Input: part model. Units: mm. Frame: model coordinates. A direction names the side the tool comes from. Coordinates: 2 decimals unless noted, no trailing zeros. Loops run counter-clockwise (first coordinate to the right, second up) from the corner with the lowest first, then second, coordinate; pieces in that order, holes last. Notation, with made-up numbers: (57, -3) -> (112, -3) arc R8 ccw to (112, 3) -> close; hole circle Ø6 at (77.25, 87.25). An arc over 180 degrees is marked (long way). Answer as a JSON object with one key per item and string values.
from build123d import *

# Parameters (mm, degrees)
SKETCH1_W               = 90
SKETCH1_H               = 110
BOSS_EXTRUDE2_DEPTH     = 6
SKETCH4_W               = 102
SKETCH4_H               = 122
SKETCH4_W_2             = 90
SKETCH4_H_2             = 110
BOSS_EXTRUDE3_DEPTH     = 55
SKETCH6_W               = 81.2
SKETCH6_H               = 58
SKETCH6_W_2             = 77.2
SKETCH6_H_2             = 54
BOSS_EXTRUDE4_DEPTH     = 4
CUT_EXTRUDE1_DEPTH      = 4
SKETCH12_W              = 77.2
SKETCH12_H              = 54
BOSS_EXTRUDE5_DEPTH     = 2
CUT_EXTRUDE2_REACH      = 165.966
FILLET1_R               = 2
FILLET2_R               = 2
FILLET3_R               = 2
BOSS_EXTRUDE7_DEPTH     = 4
SKETCH14_R              = 1.4
CUT_EXTRUDE3_DEPTH      = 8
MIRROR2_COPY_1_SKETCH_R = 1.4
MIRROR2_COPY_1_DEPTH    = 8


with BuildPart() as part:
    # Sketch1 → Boss-Extrude2 (new body)
    with BuildSketch(Plane(origin=(0, 0, 0), x_dir=(1, 0, 0), z_dir=(0, 1, 0))):
        with Locations((-45, 55)):
            Rectangle(SKETCH1_W, SKETCH1_H)
    extrude(amount=BOSS_EXTRUDE2_DEPTH)

    # Sketch4 → Boss-Extrude3 (add)
    with BuildSketch(Plane.XZ):
        with Locations((-45, -55)):
            Rectangle(SKETCH4_W, SKETCH4_H)
        with Locations((-45, -55)):
            Rectangle(SKETCH4_W_2, SKETCH4_H_2, mode=Mode.SUBTRACT)
    extrude(amount=-BOSS_EXTRUDE3_DEPTH)

    # Sketch6 → Boss-Extrude4 (add)
    with BuildSketch(Plane(origin=(0, 6, 0), x_dir=(1, 0, 0), z_dir=(0, 1, 0))):
        with Locations((-45, 77)):
            Rectangle(SKETCH6_W, SKETCH6_H)
        with Locations((-45, 77)):
            Rectangle(SKETCH6_W_2, SKETCH6_H_2, mode=Mode.SUBTRACT)
    extrude(amount=BOSS_EXTRUDE4_DEPTH)

    # Sketch11 → Cut-Extrude1 (cut)
    with BuildSketch(Plane(origin=(0, 10, 0), x_dir=(1, 0, 0), z_dir=(0, 1, 0))):
        Polygon((-6.4, 106), (-6.4, 104), (-6.4, 50), (-6.4, 48), (-4.4, 48), (-4.4, 106), align=None)
    extrude(amount=-CUT_EXTRUDE1_DEPTH, mode=Mode.SUBTRACT)

    # Sketch12 → Boss-Extrude5 (add)
    with BuildSketch(Plane(origin=(0, 6, 0), x_dir=(1, 0, 0), z_dir=(0, 1, 0))):
        with Locations((-45, 77)):
            Rectangle(SKETCH12_W, SKETCH12_H)
    extrude(amount=BOSS_EXTRUDE5_DEPTH)

    # Sketch10 → Cut-Extrude2 (cut, up to next)
    with BuildSketch(Plane(origin=(6, 0, 0), x_dir=(0, 0, -1), z_dir=(1, 0, 0)), mode=Mode.PRIVATE) as cut_extrude2_sk1:
        Polygon((92.5, 8), (104, 8), (104, 20.5), (92.5, 20.5), (92.5, 13.5), align=None)
    cut_extrude2_tool1 = extrude(cut_extrude2_sk1.sketch, amount=-CUT_EXTRUDE2_REACH, mode=Mode.PRIVATE) & part.part
    # Sketch10 → Cut-Extrude2 (cut, up to next)
    with BuildSketch(Plane(origin=(6, 0, 0), x_dir=(0, 0, -1), z_dir=(1, 0, 0)), mode=Mode.PRIVATE) as cut_extrude2_sk2:
        Polygon((82.5, 8), (92.5, 8), (92.5, 13.5), (82.5, 13.5), (82.5, 11.241721358), align=None)
    cut_extrude2_tool2 = extrude(cut_extrude2_sk2.sketch, amount=-CUT_EXTRUDE2_REACH, mode=Mode.PRIVATE) & part.part
    # Sketch10 → Cut-Extrude2 (cut, up to next)
    with BuildSketch(Plane(origin=(6, 0, 0), x_dir=(0, 0, -1), z_dir=(1, 0, 0)), mode=Mode.PRIVATE) as cut_extrude2_sk3:
        Polygon((65, 13.5), (65, 8), (75, 8), (75, 11.241721358), (75, 13.5), align=None)
    cut_extrude2_tool3 = extrude(cut_extrude2_sk3.sketch, amount=-CUT_EXTRUDE2_REACH, mode=Mode.PRIVATE) & part.part
    add(cut_extrude2_tool1.solids().sort_by_distance((6, 14.25, -98.25))[0], mode=Mode.SUBTRACT)
    add(cut_extrude2_tool2.solids().sort_by_distance((6, 10.75, -87.5))[0], mode=Mode.SUBTRACT)
    add(cut_extrude2_tool3.solids().sort_by_distance((6, 10.75, -70))[0], mode=Mode.SUBTRACT)

    # Fillet1
    fillet1_edges = [part.edges().sort_by_distance(p)[0] for p in [
        (6, 17, -92.5),
        (6, 13.5, -87.5),
        (6, 10.75, -82.5),
        (6, 8, -93.25),
        (6, 14.25, -104),
        (6, 20.5, -98.25),
        (6, 10.75, -65),
        (6, 8, -70),
        (6, 10.75, -75),
        (6, 13.5, -70),
    ]]
    fillet(fillet1_edges, radius=FILLET1_R)

    # Fillet2
    fillet2_edges = [part.edges().sort_by_distance(p)[0] for p in [
        (-96, 27.5, -116),
        (-96, 27.5, 6),
        (6, 27.5, 6),
        (6, 27.5, -116),
    ]]
    fillet(fillet2_edges, radius=FILLET2_R)

    # Fillet3
    fillet3_edges = [part.edges().sort_by_distance(p)[0] for p in [
        (0, 30.5, 0),
        (0, 30.5, -110),
        (-90, 30.5, -110),
        (-90, 30.5, 0),
    ]]
    fillet(fillet3_edges, radius=FILLET3_R)

    # Sketch13 → Boss-Extrude7 (add)
    with BuildSketch(Plane(origin=(0, 8, 0), x_dir=(1, 0, 0), z_dir=(0, 1, 0))):
        with BuildLine():
            ThreePointArc((-77.35, 96), (-77.862563133, 97.237436867), (-79.1, 97.75))
            Line((-79.1, 97.75), (-79.1, 96))
            Line((-79.1, 96), (-80.85, 96))
            ThreePointArc((-80.85, 96), (-79.1, 94.25), (-77.35, 96))
        make_face()
        with BuildLine():
            Line((-79.1, 96), (-79.1, 97.75))
            ThreePointArc((-79.1, 97.75), (-80.337436867, 97.237436867), (-80.85, 96))
            Line((-80.85, 96), (-79.1, 96))
        make_face()
        with BuildLine():
            ThreePointArc((-18.6, 52.25), (-17.362563133, 52.762563133), (-16.85, 54))
            Line((-16.85, 54), (-18.6, 54))
            Line((-18.6, 54), (-18.6, 52.25))
        make_face()
        with BuildLine():
            Line((-18.6, 54), (-16.85, 54))
            ThreePointArc((-16.85, 54), (-19.837436867, 55.237436867), (-18.6, 52.25))
            Line((-18.6, 52.25), (-18.6, 54))
        make_face()
    extrude(amount=BOSS_EXTRUDE7_DEPTH)

    # Sketch14 → Cut-Extrude3 (cut)
    with BuildSketch(Plane(origin=(0, 55, 0), x_dir=(1, 0, 0), z_dir=(0, 1, 0))):
        with Locations(Location((-92.414213562, 112.414213562, 0), (0, 0, 270))):
            Circle(SKETCH14_R)
    cut_extrude3 = extrude(amount=-CUT_EXTRUDE3_DEPTH, mode=Mode.SUBTRACT)

    # Mirror1: Cut-Extrude3 across plane
    add(cut_extrude3.mirror(Plane.ZY.offset(45)), mode=Mode.SUBTRACT)

    # Mirror2: Cut-Extrude3 across plane
    add(cut_extrude3.mirror(Plane(origin=(0, 0, -55), x_dir=(1, 0, 0), z_dir=(0, 0, -1))), mode=Mode.SUBTRACT)

    # Mirror2 copy 1 sketch → Mirror2 copy 1 (cut)
    with BuildSketch(Plane(origin=(-90, 55, -110), x_dir=(-1, 0, 0), z_dir=(0, 1, 0))):
        with Locations(Location((-92.414213562, 112.414213562, 0), (0, 0, 270))):
            Circle(MIRROR2_COPY_1_SKETCH_R)
    extrude(amount=-MIRROR2_COPY_1_DEPTH, mode=Mode.SUBTRACT)


solid = part.part
1. Line query: line 1 along X through (y, z) = (33, -23); line 2 along Z through (x, y) = (-78.5, 24); line 3 along Y through (x, z) = (-68, -7). Output: solid intervals per line, ascending.
Reply:
{"line 1": "x = -96 to -90, 0 to 6", "line 2": "z = -116 to -110, 0 to 6", "line 3": "y = 0 to 6"}
2. Section query C-C (x = -54). Return loops of the section in (y, z).
Reply:
{"outline": "(0, -116) -> (55, -116) -> (55, -110) -> (6, -110) -> (6, -106) -> (10, -106) -> (10, -104) -> (8, -104) -> (8, -50) -> (10, -50) -> (10, -48) -> (6, -48) -> (6, 0) -> (55, 0) -> (55, 6) -> (0, 6) -> close"}
3. Pin query (flat end, axial travel): P1, Ø5, axis at x = -18, z = -34.5, coming from the +Y side; P2, Ø2, axis at y = 8.5, z = -70.5, coming from the +X side; P3, Ø1, axis at x = -17.5, z = -53.5, coming from the +Y side. Return the tip coordinate at first contact, or that it passes through.
Reply:
{"P1": "stops at y = 6", "P2": "stops at x = 5.32", "P3": "stops at y = 12"}
4. Mould query, pull axis X, two halves, no side actions, for faces 1 (the face through (2, 14, -104)), 2 (the face through (-96, 27, -56)), 3 (the face through (-47, 8, -48)). Classes: pulls with the +X half, pulls with the -X half, needs draft (parallel to the pull), parting line crosses it, or undercut.
Reply:
{"face 1": "needs draft", "face 2": "pulls with the -X half", "face 3": "undercut"}
5. Section query A-A (z = -71.5). Return loops of the section in (x, y), plus the area to 3 significant figures.
Reply:
{"outline": "(-96, 0) -> (6, 0) -> (6, 6) arc R2 ccw to (4, 8) -> (0, 8) -> (0, 6) -> (-6.4, 6) -> (-6.4, 8) -> (-83.6, 8) -> (-83.6, 10) -> (-85.6, 10) -> (-85.6, 6) -> (-90, 6) -> (-90, 55) -> (-96, 55) -> close; (0, 13.5) -> (4, 13.5) arc R2 ccw to (6, 15.5) -> (6, 55) -> (0, 55) -> close", "area": "1,330 mm2"}
6. Section query D-D (z = -100.5). Return loops of the section in (x, y).
Reply:
{"outline": "(-96, 0) -> (6, 0) -> (6, 6) arc R2 ccw to (4, 8) -> (0, 8) -> (0, 6) -> (-6.4, 6) -> (-6.4, 8) -> (-83.6, 8) -> (-83.6, 10) -> (-85.6, 10) -> (-85.6, 6) -> (-90, 6) -> (-90, 55) -> (-96, 55) -> close; (0, 20.5) -> (4, 20.5) arc R2 ccw to (6, 22.5) -> (6, 55) -> (0, 55) -> close"}
7. Access query for faces 4 (the face through (-79, 12, -96)), 5 (the face through (2, 13.5, -88)), 6 (the face through (1.99, 51.06, 1.08)). Directions: +Z, -Z, +X, -X, +Y, -Y. A direction counts if a zero-diameter tool reaches every point of the face in a straight line with its end or side. Return the directions, or none.
Reply:
{"face 4": "+X, +Y", "face 5": "+X", "face 6": "+Y"}
8. Section query B-B (y = 33.5). Return loops of the section in (x, z), plus the area to 3 significant figures.
Reply:
{"outline": "(-96, -114) arc R2 ccw to (-94, -116) -> (4, -116) arc R2 ccw to (6, -114) -> (6, 4) arc R2 ccw to (4, 6) -> (-94, 6) arc R2 ccw to (-96, 4) -> close; hole (-90, -108) arc R2 ccw to (-88, -110) -> (-2, -110) arc R2 ccw to (0, -108) -> (0, -2) arc R2 ccw to (-2, 0) -> (-88, 0) arc R2 ccw to (-90, -2) -> close", "area": "2,540 mm2"}
